Can you work these out from the model? Positions are in its coordinate system, mm. A direction names the side the tool comes from. Round coordinates to 2 decimals unless told otherwise and drop trailing zeros. Loops run counter-clockwise (first coordinate to the right, second up) from the corner with the lowest first, then second, coordinate; pieces in that order, holes last. Notation, with made-up numbers: (5.25, 46) -> (9.25, 46) arc R26 cw to (9.25, 70) -> close; hole circle Ø11 at (78, 83.5). An arc over 180 degrees is marked (long way). Write item = value, one per line.
from build123d import *


with BuildPart() as part:
    # Sketch3 → Revolve1 (revolve)
    with BuildSketch(Plane.XY, mode=Mode.PRIVATE) as revolve1_sk:
        Polygon((63.5, 139.7), (63.5, 152.4), (-63.5, 152.4), (-63.5, 139.7), (-12.7, 139.7), (-12.7, 12.7), (12.7, 12.7), (12.7, 139.7), align=None)
        with BuildLine():
            Line((-63.5, 152.4), (63.5, 152.4))
            ThreePointArc((63.5, 152.4), (82.597266275, 215.469039665), (49.79563591, 272.622013244))
            Line((49.79563591, 272.622013244), (-49.79563591, 272.622013244))
            ThreePointArc((-49.79563591, 272.622013244), (-82.597266275, 215.469039665), (-63.5, 152.4))
        make_face()
    revolve(revolve1_sk.sketch.rotate(Axis((12.7, 0, 0), (-1, 0, 0)), 90), axis=Axis((12.7, 0, 0), (-1, 0, 0)))


solid = part.part
1. We'd pull the mould along Z, two halves only. Please class faces 3 (the cylindrical face through (0.2, 7.7, 10.1)), 4 (the flat face through (63.5, 123, 67)), 5 (the cylindrical face through (-0.697, -81.888, -260.033)): released by +Z, released by -Z, zero draft, split by the parting line, or undercut.
Entries:
face_3 = undercut
face_4 = undercut
face_5 = split by the parting line
2. Suppose I cut it at C-C, the plane x = -20. List the corners of the cut face in (y, z) for me.
Entries:
outline = circle Ø545.24 at (0, 0); hole circle Ø279.4 at (0, 0)
3. Suppose I cut it at A-A, the plane z = 0. List the corners of the cut face in (x, y) for me.
Entries:
outline = (-63.5, -152.4) arc R83.13 ccw to (-49.8, -272.62) -> (49.8, -272.62) arc R83.13 ccw to (63.5, -152.4) -> (63.5, -139.7) -> (12.7, -139.7) -> (12.7, -12.7) -> (-12.7, -12.7) -> (-12.7, -139.7) -> (-63.5, -139.7) -> close; (-63.5, 139.7) -> (-12.7, 139.7) -> (-12.7, 12.7) -> (12.7, 12.7) -> (12.7, 139.7) -> (63.5, 139.7) -> (63.5, 152.4) arc R83.13 ccw to (49.8, 272.62) -> (-49.8, 272.62) arc R83.13 ccw to (-63.5, 152.4) -> close
4. For faces 1 (the flat face through (-12.7, -2, -29)), 2 (the flat face through (12.7, -2, 29)), which set-ups out of +Z, -Z, +X, -X, +Y, -Y let a thin tool reach every point of the face, with its end or its side?
Entries:
face_1 = -X
face_2 = +X
5. I'm going to push flat-ended pins straight in: pin 1 (6 mm diameter, centred on x = -4, z = -216, fed in from -Y); pin 2 (1.5 mm diameter, centred on y = -132.5, z = 16.5, fed in from +X); pin 3 (6 mm diameter, centred on y = -205, z = 5.5, fed in from +X). Where does each tip first touch, or does it pass through?
Entries:
pin_1 = -170.16
pin_2 = 12.7
pin_3 = 83.13
6. I need wall thicknesses on line 1 (Y direction, x = 36, z = 0); line 2 (X direction, y = -84.5, z = 2.5); line 3 (Y direction, x = 0, z = 0). Which ranges of each line are inside material? Lowest first, please. Write a range as [from, to].
Entries:
line_1 = [-272.62, -139.7], [139.7, 272.62]
line_2 = [-12.7, 12.7]
line_3 = [-272.62, -12.7], [12.7, 272.62]
